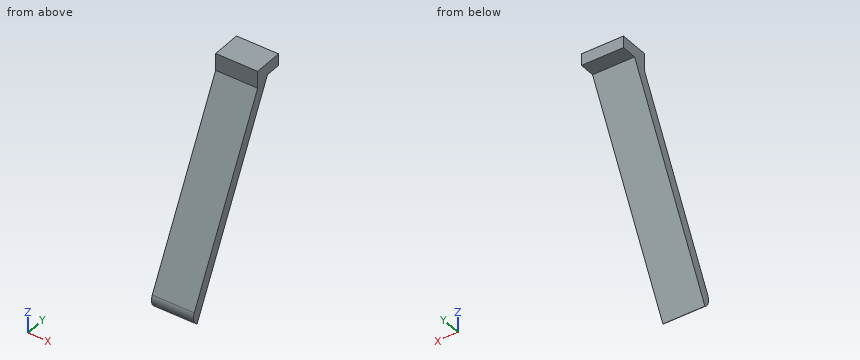
from build123d import *

# Parameters (mm, degrees)
BOSS_EXTRUDE1_DEPTH = 4.3


with BuildPart() as part:
    # Sketch1 → Boss-Extrude1 (new body)
    with BuildSketch(Plane(origin=(0, 0, 0), x_dir=(0, 0, -1), z_dir=(1, 0, 0))):
        with BuildLine():
            ThreePointArc((-11.083862383, -16.615210797), (-10.301073063, -16.690701101), (-9.678172689, -16.210645864))
            Line((-9.678172689, -16.210645864), (-29.442415971, -6.108537965))
            Line((-29.442415971, -6.108537965), (-29.442415971, -4.512715584))
            Line((-29.442415971, -4.512715584), (-30.642415971, -4.512715584))
            Line((-30.642415971, -4.512715584), (-30.642415971, -7.512715584))
            Line((-30.642415971, -7.512715584), (-28.892415971, -7.512715584))
            Line((-28.892415971, -7.512715584), (-11.083862383, -16.615210797))
        make_face()
    extrude(amount=BOSS_EXTRUDE1_DEPTH)


solid = part.part
Verification items for the finished model (mm, model axes). Coordinates: 2 decimals unless noted, no trailing zeros. Order: outer loops, then holes, each group sorted by start corner. A loop starts at its lowest first (then second) coordinate and runs counter-clockwise, first axis right, second up. Notation, with made-up numbers: (-17.75, 41) -> (1.25, 41) arc R18 ccw to (1.25, 56) -> close; hole circle Ø5 at (64, 48). An arc over 180 degrees is marked (long way). Put each result on its own line as item: value. Start each with the question number.
1. Cross-section at B-B, the plane y = -6.5. Record the boundary of the cut face in (x, z), then the cut area to 3 significant figures.
2. Cross-section at A-A, the plane x = 3.75. Record the boundary of the cut face in (y, z), then the cut area to 3 significant figures.
3. Cross-section at C-C, the plane z = 14.25. Record the boundary of the cut face in (x, y).
4. Material ranges on L1, parallel to Z at x = 0.2, y = -6; L2, parallel to Y at x = 2.2, z = 21; L3, parallel to Y at x = 3.45, z = 28.25, recorded low to high. Write a range as [from, to].
5. Go/stop test with flat-tipped pins: pin 1 Ø1.9 at (x, z) = (1.5, 30) entering from -Y; pin 2 Ø1.5 at (x, z) = (2, 27) entering from +Y; pin 3 Ø2 at (x, y) = (1.5, -12.5) entering from -Z. Record where each tip stops, or that it passes through.
Computed:
1. outline: (0, 28.68) -> (4.3, 28.68) -> (4.3, 30.64) -> (0, 30.64) -> close
1. area: 8.45 mm2
2. outline: (-16.62, 11.08) arc R1.07 ccw to (-16.21, 9.68) -> (-6.11, 29.44) -> (-4.51, 29.44) -> (-4.51, 30.64) -> (-7.51, 30.64) -> (-7.51, 28.89) -> close
2. area: 25.4 mm2
3. outline: (0, -15) -> (4.3, -15) -> (4.3, -13.87) -> (0, -13.87) -> close
4. L1: [29.44, 30.64]
4. L2: [-11.55, -10.42]
4. L3: [-7.84, -6.72]
5. pin 1: y = -7.51
5. pin 2: y = -6.97
5. pin 3: z = 14.98
